Check sheet for the modelled part. Datum: model origin and axes. Units: mm. Face numbers are marked on the shaded views. A direction names the side the tool comes from. Coordinates: 2 decimals unless noted, no trailing zeros. Write each loop counter-clockwise with the first axis right and the second up, starting at its lowest first coordinate (ties: lowest second). Pieces come first, ordered by that corner, then holes. Notation, with made-up numbers: M 32,15 L 79,15 A17 ccw 79,20 Z; hole C 2,9 d8. An arc over 180 degrees is marked long. Answer as CSV lines item,"result".
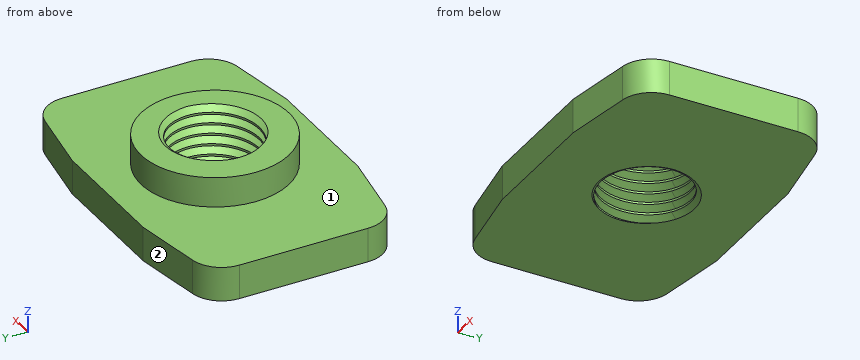
from build123d import *

# Parameters (mm, degrees)
BOSS_EXTRUDE1_DEPTH        = 1.6
DRAFT1_ANGLE               = 9.10617604
SKETCH2_W                  = 3.45
SKETCH2_H                  = 1.4
F_4_2_4_2_DIAMETER_HOLE1_D = 4.2
FILLET1_R                  = 1.5
CUT_SWEEP1_PITCH           = 0.5


with BuildPart() as part:
    # Sketch1 → Boss-Extrude1 (new body)
    with BuildSketch(Plane.XY.offset(1.6)):
        Polygon((3, -5), (6.092206474, -4.504366896), (7.5, 4.278719262), (3, 5), (-3, 5), (-7.5, 4.278719262), (-7.5, -4.278719262), (-3, -5), align=None)
    extrude(amount=-BOSS_EXTRUDE1_DEPTH)

    # Draft1
    draft1_faces = [part.faces().sort_by_distance(p)[0] for p in [
        (6.796103237, -0.112823817, 0.8),
    ]]
    draft(draft1_faces, Plane(origin=(7.5, 4.278719262, 0), x_dir=(0.9873967528040769, -0.15826450186938548, 0), z_dir=(0.15826450186938548, 0.9873967528040769, 0)), DRAFT1_ANGLE)

    # Sketch2 → Revolve1 (revolve)
    with BuildSketch(Plane.XZ, mode=Mode.PRIVATE) as revolve1_sk:
        with Locations((1.725, 2.3)):
            Rectangle(SKETCH2_W, SKETCH2_H)
    revolve(revolve1_sk.sketch.rotate(Axis((0, 0, 3), (0, 0, -1)), 180), axis=Axis((0, 0, 3), (0, 0, -1)))

    # Ø4.2 (4.2) Diameter Hole1 (through all)
    with Locations(Plane.XY.offset(3)):
        with Locations((0, 0)):
            Hole(F_4_2_4_2_DIAMETER_HOLE1_D / 2)

    # Fillet1
    fillet1_edges = [part.edges().sort_by_distance(p)[0] for p in [
        (-7.5, -4.278719262, 0.8),
        (-7.5, 4.278719262, 0.8),
        (7.5, 4.278719262, 0.8),
        (7.5, -4.278719262, 0.8),
    ]]
    fillet(fillet1_edges, radius=FILLET1_R)

    # Cut-Sweep1: arcs per turn and ends read off the stored shape
    # Cut-Sweep1: the profile of Sketch6 screwed along a right-hand helix through 8 turns, 6 arcs to a turn; built about Z, then put on its axis
    cut_sweep1_z = Axis((0, 0, 0), (0, 0, 1))
    cut_sweep1_corners = [(-1.223205081, -2.118653348, -0.666666667), (-0.96339746, -1.668653348, -0.366666667), (-0.96339746, -1.668653348, -0.966666667)]
    with BuildLine(mode=Mode.PRIVATE) as cut_sweep1_profile:
        Line(cut_sweep1_corners[0], cut_sweep1_corners[1])
        Line(cut_sweep1_corners[1], cut_sweep1_corners[2])
        Line(cut_sweep1_corners[2], cut_sweep1_corners[0])
    cut_sweep1_cap = Face(cut_sweep1_profile.wire())
    cut_sweep1_turn_angles = [0, 30, 60, 90, 120, 150, 180, 210, 240, 270, 300, 330, 360]
    cut_sweep1_turn_weights = [1, 0.8660254037844387, 1, 0.8660254037844387, 1, 0.8660254037844387, 1, 0.8660254037844387, 1, 0.8660254037844387, 1, 0.8660254037844387, 1]
    cut_sweep1_turn_rails = [Edge.make_bspline([Vector(p[0], p[1], 0).rotate(cut_sweep1_z, cut_sweep1_turn_angles[k]) / cut_sweep1_turn_weights[k] + Vector(0, 0, p[2] + CUT_SWEEP1_PITCH * cut_sweep1_turn_angles[k] / 360) for k in range(13)], [0, 0, 0, 1, 1, 2, 2, 3, 3, 4, 4, 5, 5, 6, 6, 6], 2, cut_sweep1_turn_weights) for p in cut_sweep1_corners]
    cut_sweep1_turn_sides = [Face.make_surface_from_curves(cut_sweep1_turn_rails[p[0]], cut_sweep1_turn_rails[p[1]]) for p in [(0, 1), (1, 2), (2, 0)]]
    cut_sweep1 = Plane(origin=(0, 0, 3), x_dir=(1, 0, 0), z_dir=(0, 0, -1)) * Solid(Shell([*[p.moved(Location((0, 0, CUT_SWEEP1_PITCH * i))) for i in range(8) for p in cut_sweep1_turn_sides], cut_sweep1_cap, cut_sweep1_cap.rotate(cut_sweep1_z, 2880).moved(Location((0, 0, CUT_SWEEP1_PITCH * 2880 / 360)))]))
    add(cut_sweep1, mode=Mode.SUBTRACT)


solid = part.part
1) Thickness scan on line 1 along Y through (x, z) = (0, 1.2); line 2 along Z through (x, y) = (0.75, -4.5); line 3 along Y through (x, z) = (0, 1.35). Record the ranges inside material, lowest first.
Answer key:
line 1,"y = -5 to -2.14, 2.32 to 5"
line 2,"z = 0 to 1.6"
line 3,"y = -5 to -2.4, 2.1 to 5"
2) Tool access check on the marked faces 1 and 2. Record the directions out of +Z, -Z, +X, -X, +Y, -Y that give a thin tool (end or side, any length) a straight path to the whole face; none if there is none.
Answer key:
face 1,"+Z"
face 2,"+Z, -Z, -X, +Y"
3) Section check C-C, the plane x = -6.5. Record the boundary of the cut face in (y, z).
Answer key:
outline,"M -4.41,0 L 4.41,0 L 4.41,1.6 L -4.41,1.6 Z"
4) Section check D-D, the plane x = 5.75. Record the boundary of the cut face in (y, z).
Answer key:
outline,"M -4.56,0 L 4.56,0 L 4.56,1.6 L -4.56,1.6 Z"
5) Section check A-A, the plane x = 2.25. Give the number of separate pieces and of enclosed holes in the cut face, plus the area to 3 significant figures.
Answer key:
separate pieces,"1"
enclosed holes,"5"
area,"21.6 mm2"
6) Section check B-B, the plane x = -3.25. Record the boundary of the cut face in (y, z).
Answer key:
outline,"M -4.96,0 L 4.96,0 L 4.96,1.6 L 1.16,1.6 L 1.16,3 L -1.16,3 L -1.16,1.6 L -4.96,1.6 Z"
7) Depth check by flat-ended pin: P1, Ø1, axis at x = 5, z = 0.5, coming from the -Y side; P2, Ø6, axis at x = -1.5, y = -1.5, coming from the -Z side; P3, Ø1, axis at x = -5.5, y = 3.5, coming from the +Z side. Enter the tip coordinate at first touch or a pass-through.
Answer key:
P1,"stops at y = -4.76"
P2,"stops at z = 0"
P3,"stops at z = 1.6"
